Here's the drawing with two shaded views (mm, measured from the low corner). I have some questions. Round coordinates to 2 decimals unless told otherwise and drop trailing zeros. Order: outer loops, then holes, each group sorted by start corner. A loop starts at its lowest first (then second) coordinate and runs counter-clockwise, first axis right, second up.
Q1. If we section it at B-B (x = 80.5): Please give me the cut outline in (y, z).
Q2. Will these pins go through, and if not, where does the flat tip stop? P1, Ø0.9, axis at x = 2, z = 1, coming from the -Y side; P2, Ø0.9, axis at x = 43, z = 1, coming from the -Y side; P3, Ø0.9, axis at y = 1.5, z = 1.5, coming from the -X side.
Q3. If I drill on line 1 (X direction, y = 56, z = 0.4); line 2 (Y direction, x = 41.5, z = 0.4), over which ranges is the centre line in solid material (lowest first)?
Q4. If we section it at C-C (y = 35): Please give me the cut outline in (x, z).
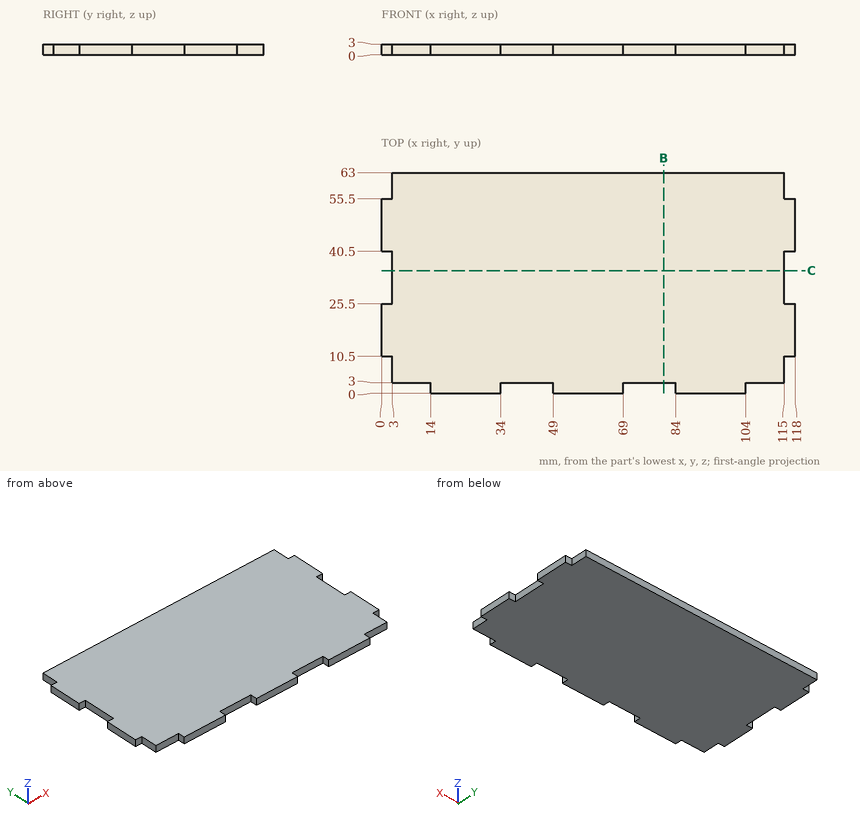
Solution:
1. outline: (3, 0) - (63, 0) - (63, 3) - (3, 3) - close
2. P1: stops at y = 10.5
2. P2: stops at y = 3
2. P3: stops at x = 14
3. line 1: x = 3 to 115
3. line 2: y = 3 to 63
4. outline: (3, 0) - (115, 0) - (115, 3) - (3, 3) - close
